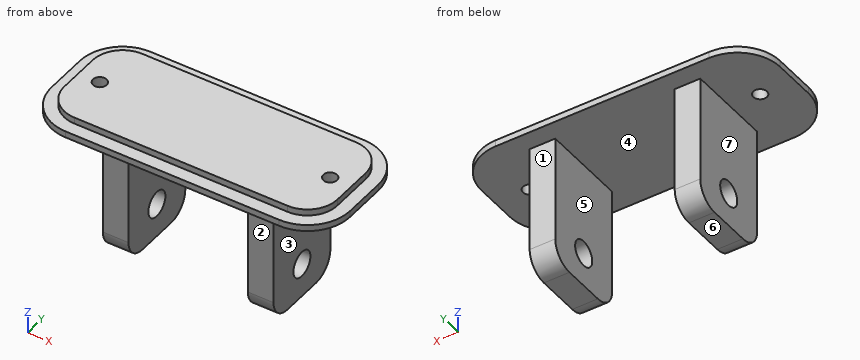
Autodesk Inventor part; units mm, degrees
ref_plane "YZ Plane" through (0, 0, 0) normal (1, 0, 0) x (0, 1, 0)
ref_plane "XZ Plane" through (0, 0, 0) normal (0, 1, 0) x (-1, 0, 0)
ref_plane "XY Plane" through (0, 0, 0) normal (0, 0, 1) x (1, 0, 0)
sketch "Sketch1" plane through (0, 0, 0) normal (0, 0, 1) x (1, 0, 0)
  line L0 (-35, 15) -> (35, 15)
  line L1 (35, 15) -> (35, -15)
  line L2 (35, -15) -> (-35, -15)
  line L3 (-35, -15) -> (-35, 15)
  point P0 (0, 0)
  dimension "d0" = 70
  dimension "d1" = 30
  dimension "d7" = 35
  dimension "d8" = 15
extrude "Extrusion1" add sketch "Sketch1" along normal blind 3
fillet "Fillet1" radius 10 4 edges at (-35, 15, 1.5) (-35, -15, 1.5) (35, -15, 1.5) (35, 15, 1.5)
sketch "Sketch6" plane through (0, 0, 3) normal (0, 0, 1) x (1, 0, 0)
  arc A0 (35, 5) -> (25, 15) centre (25, 5) ccw
  line L0 (25, 15) -> (-25, 15)
  arc A1 (-25, 15) -> (-35, 5) centre (-25, 5) ccw
  line L1 (-35, 5) -> (-35, -5)
  arc A2 (-35, -5) -> (-25, -15) centre (-25, -5) ccw
  line L2 (-25, -15) -> (25, -15)
  arc A3 (25, -15) -> (35, -5) centre (25, -5) ccw
  line L3 (35, -5) -> (35, 5)
  arc A4 (-25, 12) -> (-32, 5) centre (-25, 5) ccw
  line L4 (-25, 12) -> (25, 12)
  arc A5 (32, 5) -> (25, 12) centre (25, 5) ccw
  line L5 (32, 5) -> (32, -5)
  arc A6 (25, -12) -> (32, -5) centre (25, -5) ccw
  line L6 (25, -12) -> (-25, -12)
  arc A7 (-32, -5) -> (-25, -12) centre (-25, -5) ccw
  line L7 (-32, -5) -> (-32, 5)
  point P0 (0, 0)
  dimension "d43" = 3
extrude "Extrusion5" cut sketch "Sketch6" against normal blind 1.5
sketch "Sketch7" plane through (0, 0, 3) normal (0, 0, 1) x (1, 0, 0)
  line L0 (-35, -5) -> (-35, 5)
  line L1 (35, 5) -> (35, -5)
  circle A0 centre (-27, 0) radius 1.6
  circle A1 centre (27, 0) radius 1.6
  point P0 (0, 0)
  point P1 (-35, 0)
  dimension "d46" = 3.2
  dimension "d47" = 8
  dimension "d48" = 3.2
  dimension "d49" = 8
extrude "Extrusion6" cut sketch "Sketch7" against normal through all
sketch "Sketch8" plane through (0, 0, 0) normal (0, 0, -1) x (-1, 0, 0)
  line L0 (-20, 10.5653) -> (-14, 10.5653)
  line L1 (-14, 10.5653) -> (-14, -9.4347)
  line L2 (-14, -9.4347) -> (-20, -9.4347)
  line L3 (-20, -9.4347) -> (-20, 10.5653)
  line L4 (14, 10.5653) -> (20, 10.5653)
  line L5 (20, 10.5653) -> (20, -9.4347)
  line L6 (20, -9.4347) -> (14, -9.4347)
  line L7 (14, -9.4347) -> (14, 10.5653)
  line L8 (-35, -5) -> (-35, 5)
  line L9 (35, 5) -> (35, -5)
  point P0 (0, 0)
  point P1 (-35, 0)
  dimension "d52" = 20
  dimension "d53" = 6
  dimension "d54" = 6
  dimension "d55" = 15
  dimension "d56" = 15
extrude "Extrusion7" add sketch "Sketch8" along normal blind 30
sketch "Sketch9" plane through (20, -9.4347, 0) normal (1, 0, 0) x (0, 0, -1)
  circle A0 centre (22, 10) radius 3
  line L0 (0, 0) -> (30, 0)
  line L1 (30, 20) -> (30, 0)
  point P0 (0, 9.4347)
  dimension "d59" = 6
  dimension "d60" = 10
  dimension "d61" = 8
extrude "Extrusion8" cut sketch "Sketch9" against normal through all
fillet "Fillet2" radius 5 4 edges at (17, -9.4347, -30) (17, 10.5653, -30) (-17, 10.5653, -30) (-17, -9.4347, -30)
properties part number "sensor_cover_ultrasonic_2"
For this review, take the finished solid that the model builds, in its own axes (mm). Face numbers are marked on the shaded views. A direction names the side the tool comes from. Round coordinates to 2 decimals unless told otherwise and drop trailing zeros. Order: outer loops, then holes, each group sorted by start corner. A loop starts at its lowest first (then second) coordinate and runs counter-clockwise, first axis right, second up. Notation, with made-up numbers: M -2,13 L 34,13 A17 cw 34,37 Z; hole C -12,40.25 d10. An arc over 180 degrees is marked long. Write each question's results on one line, items separated by ' | '. Start each with the question number.
1. Add section C-C (x = 15.5). State the section outline as (y, z) points, then the cut area to 3 significant figures.
2. Tool access review of the marked faces 1, 2 and 3: name each direction out of +Z, -Z, +X, -X, +Y, -Y from which nothing blocks a thin tool from reaching the whole face with its end or side.
3. Add section D-D (x = -27). State the section outline as (y, z) points.
4. To check wall thickness, follow L1, parallel to X at y = -8.75, z = -22; L2, parallel to Y at x = -16.25, z = -22; L3, parallel to Z at x = 29.5, y = -7. State the ranges of each line that lie inside material, in increasing order. Write a range as [from, to].
5. Draft analysis for pull direction X (two halves, no side actions). For the marked faces 4, 5, 6 and 7, state which applies: pulls with the +X half, pulls with the -X half, needs draft (parallel to the pull), parting line crosses it, or undercut.
6. Clearance check with flat-ended pins moving along their axes: pin 1 Ø2 at (y, z) = (-9.5, -0.5) entering from -X; pin 2 Ø10 at (y, z) = (-0.5, -21.5) entering from -X; pin 3 Ø3 at (x, z) = (16.5, -12.5) entering from -Y. State where each tip first meets the part, or that it passes through.
7. Add section B-B (z = -22). State the section outline as (x, y) points, then the cut area to 3 significant figures.
8. Add section A-A (z = -2.5). State the section outline as (x, y) points.
Output values:
1) outline: M -15,0 L -9.43,0 L -9.43,-25 A5 ccw -4.43,-30 L 5.57,-30 A5 ccw 10.57,-25 L 10.57,0 L 15,0 L 15,1.5 L 12,1.5 L 12,3 L -12,3 L -12,1.5 L -15,1.5 Z; hole C 0.57,-22 d6 | area: 642 mm^2
2) face 1: -Z, +X, -X, +Y | face 2: -Z, +X, -X, -Y | face 3: -Z, +X, +Y, -Y
3) outline: M -14.8,0 L -1.6,0 L -1.6,3 L -11.71,3 L -11.71,1.5 L -14.8,1.5 Z; M 1.6,0 L 14.8,0 L 14.8,1.5 L 11.71,1.5 L 11.71,3 L 1.6,3 Z
4) L1: [-20, -14], [14, 20] | L2: [-9.43, -2.43], [3.57, 10.57] | L3: [0, 3]
5) face 4: undercut | face 5: undercut | face 6: needs draft | face 7: pulls with the -X half
6) pin 1: x = -34.32 | pin 2: x = -20 | pin 3: y = -9.43
7) outline: M -20,-9.43 L -14,-9.43 L -14,-2.43 L -20,-2.43 Z; M -20,3.57 L -14,3.57 L -14,10.57 L -20,10.57 Z; M 14,-9.43 L 20,-9.43 L 20,-2.43 L 14,-2.43 Z; M 14,3.57 L 20,3.57 L 20,10.57 L 14,10.57 Z | area: 168 mm^2
8) outline: M -20,-9.43 L -14,-9.43 L -14,10.57 L -20,10.57 Z; M 14,-9.43 L 20,-9.43 L 20,10.57 L 14,10.57 Z
